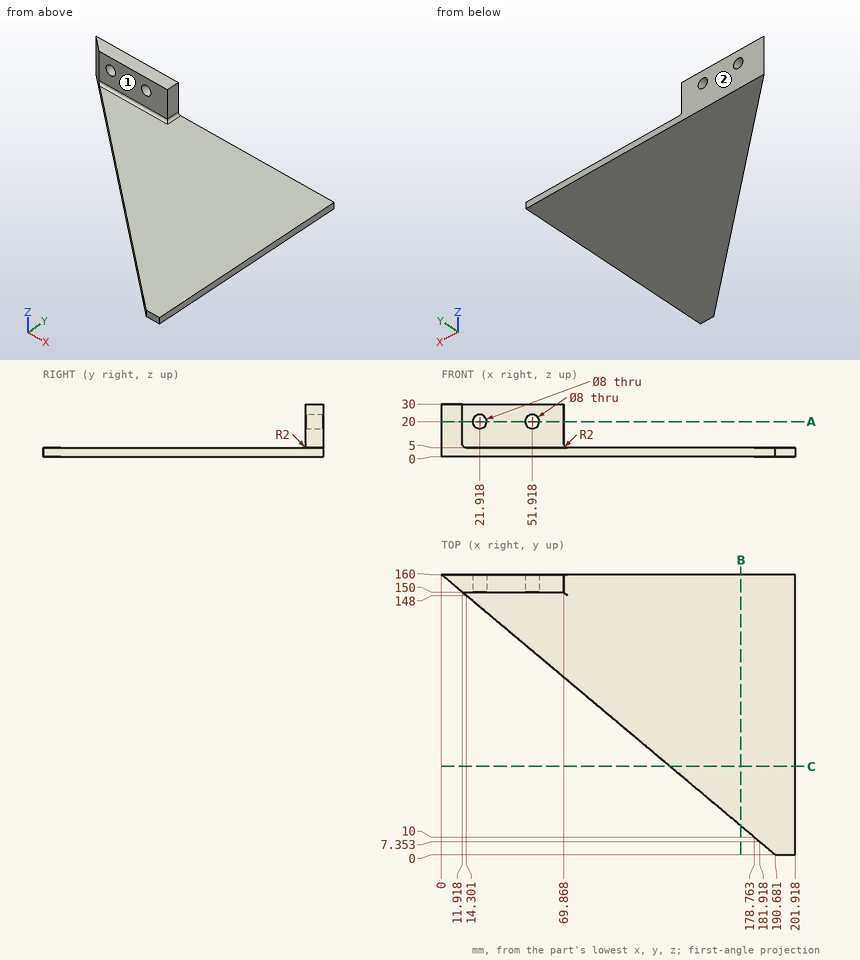
Can you work these out from the drawing? Everything is in mm from the part's minimum corner. A direction names the side the tool comes from. Round coordinates to 2 decimals unless told otherwise and drop trailing zeros. Order: outer loops, then holes, each group sorted by start corner. A loop starts at its lowest first (then second) coordinate and runs counter-clockwise, first axis right, second up.
(1) If we section it at C-C (y = 50.5): Please give me the cut outline in (x, z), plus the area to 3 significant figures.
Results are:
outline: (130.5, 0) - (201.92, 0) - (201.92, 5) - (130.5, 5) - close
area: 357 mm2
(2) I'm going to push flat-ended pins straight in: pin 1 (10 mm diameter, centred on x = 139, y = 96.5, fed in from +Z); pin 2 (5 mm diameter, centred on y = 155, z = 15.5, fed in from +X); pin 3 (13 mm diameter, centred on x = 51.92, z = 20, fed in from -Y). Where does each tip first touch, or does it pass through?
Results are:
pin 1: stops at z = 5
pin 2: stops at x = 69.87
pin 3: stops at y = 150
(3) If we section it at B-B (x = 171): Please give me the cut outline in (y, z).
Results are:
outline: (16.51, 0) - (160, 0) - (160, 5) - (16.51, 5) - close
(4) If I drill on L1, parallel to X at y = 157, z = 20 (1 decimal); L2, parallel to Z at x = 35, y = 145; L3, parallel to X at y = 158.25, z = 20 (1 decimal), over which ranges is the centre line in solid material (lowest first)?
Results are:
L1: x = 3.6 to 17.9, 25.9 to 47.9, 55.9 to 69.9
L2: z = 0 to 5
L3: x = 2.1 to 17.9, 25.9 to 47.9, 55.9 to 69.9
(5) If we section it at A-A (z = 20): Please give me the cut outline in (x, y), plus the area to 3 significant figures.
Results are:
outline: (0, 160) - (11.92, 150) - (17.92, 150) - (17.92, 160) - close; (25.92, 150) - (47.92, 150) - (47.92, 160) - (25.92, 160) - close; (55.92, 150) - (69.87, 150) - (69.87, 160) - (55.92, 160) - close
area: 479 mm2
(6) On a 3-axis mill with a long thin cutter (end or side, diameter ignored), from which of +Z, -Z, +X, -X, +Y, -Y can I reach the whole of each face in a straight line? I mean the marked faces 1 and 2. Say none if no direction works.
Results are:
face 1: +Z, +X, -X, -Y
face 2: +Z, -Z, +X, -X, +Y
